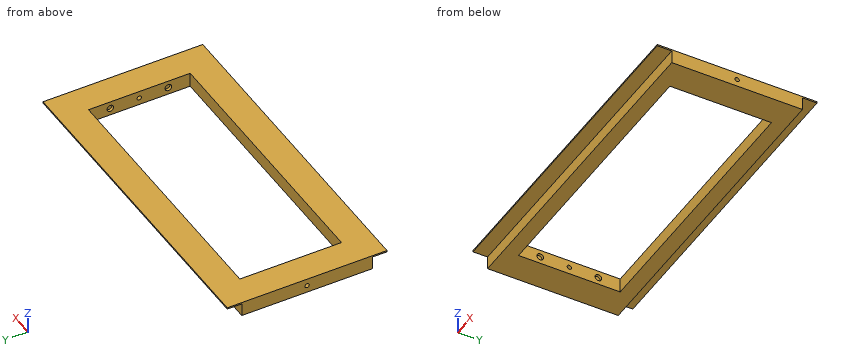
from build123d import *

# Parameters (mm, degrees)
F0_W      = 284.48
F0_H      = 139.7
F1_DEPTH  = 12.7
F2_W      = 233.68
F2_H      = 88.9
F3_DEPTH  = 25.4
F4_R      = 1.905
F5_DEPTH  = 508
F6_R      = 2.921
F7_DEPTH  = 2.5019
F8_R      = 2.921
F9_DEPTH  = 2.5019
F10_W     = 12.7
F10_H     = 11.43
F11_DEPTH = 508
F12_W     = 12.7
F12_H     = 11.43
F13_DEPTH = 508


with BuildPart() as f1:
    # F0 (on Top) → F1 (new body)
    with BuildSketch(Plane.XY):
        Rectangle(F0_W, F0_H)
    extrude(amount=F1_DEPTH)

    # F2 (on face) → F3 (cut)
    with BuildSketch(Plane.XY.offset(12.7)):
        Rectangle(F2_W, F2_H)
    extrude(amount=-F3_DEPTH, mode=Mode.SUBTRACT)

    # F4 (on face) → F5 (cut)
    with BuildSketch(Plane(origin=(-142.24, 0, 0), x_dir=(0, -1, 0), z_dir=(-1, 0, 0))):
        with Locations((0, 6.35)):
            Circle(F4_R)
    extrude(amount=-F5_DEPTH, mode=Mode.SUBTRACT)

    # F6 (on face) → F7 (cut)
    with BuildSketch(Plane.YZ.offset(-116.84)):
        with Locations((-25.4, 6.35)):
            Circle(F6_R)
        with Locations((25.4, 6.35)):
            Circle(F6_R)
    extrude(amount=-F7_DEPTH, mode=Mode.SUBTRACT)

    # F8 (on face) → F9 (cut)
    with BuildSketch(Plane(origin=(116.84, 0, 0), x_dir=(0, -1, 0), z_dir=(-1, 0, 0))):
        with Locations((-25.4, 6.35)):
            Circle(F8_R)
        with Locations((25.4, 6.35)):
            Circle(F8_R)
    extrude(amount=-F9_DEPTH, mode=Mode.SUBTRACT)

    # F10 (on face) → F11 (cut)
    with BuildSketch(Plane.YZ.offset(142.24)):
        with Locations((-63.5, 5.715)):
            Rectangle(F10_W, F10_H)
    extrude(amount=-F11_DEPTH, mode=Mode.SUBTRACT)

    # F12 (on face) → F13 (cut)
    with BuildSketch(Plane.YZ.offset(142.24)):
        with Locations((63.5, 5.715)):
            Rectangle(F12_W, F12_H)
    extrude(amount=-F13_DEPTH, mode=Mode.SUBTRACT)


solid = f1.part
Geometry check sheet. Reference: the model listing, model coordinates, mm. Give positions to 0.01 mm unless a question says otherwise; leave off trailing zeros. Write each loop counter-clockwise with the first axis right and the second up, starting at its lowest first coordinate (ties: lowest second). Pieces come first, ordered by that corner, then holes.
1) Cross-section at C-C (y = -15.5). Record the boundary of the cut face in (x, z), plus the area to 3 significant figures.
Values follow:
outline: (-142.24, 0) - (-116.84, 0) - (-116.84, 12.7) - (-142.24, 12.7) - close; (116.84, 0) - (142.24, 0) - (142.24, 12.7) - (116.84, 12.7) - close
area: 645 mm2
2) Thickness scan on line 1 (Y direction, x = 55, z = 4.75); line 2 (X direction, y = -12.5, z = 8.75); line 3 (Z direction, x = 118, y = 25). Record the ranges inside material, lowest first.
Values follow:
line 1: y = -57.15 to -44.45, 44.45 to 57.15
line 2: x = -142.24 to -116.84, 116.84 to 142.24
line 3: z = 0 to 3.46, 9.24 to 12.7
3) Go/stop test with flat-tipped pins: pin 1 Ø12 at (x, y) = (-112, 4.5) entering from -Z; pin 2 Ø4 at (x, y) = (-22, 66.5) entering from -Z; pin 3 Ø1.5 at (x, z) = (1.5, 10) entering from +Y; pin 4 Ø5.5 at (x, z) = (-66.5, 4.5) entering from -Y. Record where each tip stops, or that it passes through.
Values follow:
pin 1: stops at z = 0
pin 2: stops at z = 11.43
pin 3: stops at y = 57.15
pin 4: stops at y = -57.15
4) Cross-section at A-A (y = 25.4). Record the boundary of the cut face in (x, z).
Values follow:
outline: (-142.24, 0) - (-116.84, 0) - (-116.84, 3.43) - (-119.34, 3.43) - (-119.34, 9.27) - (-116.84, 9.27) - (-116.84, 12.7) - (-142.24, 12.7) - close; (116.84, 0) - (142.24, 0) - (142.24, 12.7) - (116.84, 12.7) - (116.84, 9.27) - (119.34, 9.27) - (119.34, 3.43) - (116.84, 3.43) - close
5) Cross-section at B-B (x = 84.5). Record the boundary of the cut face in (y, z), plus the area to 3 significant figures.
Values follow:
outline: (-69.85, 11.43) - (-57.15, 11.43) - (-57.15, 0) - (-44.45, 0) - (-44.45, 12.7) - (-69.85, 12.7) - close; (44.45, 0) - (57.15, 0) - (57.15, 11.43) - (69.85, 11.43) - (69.85, 12.7) - (44.45, 12.7) - close
area: 355 mm2
